```python
from build123d import *

# Parameters (mm, degrees)
F1_DEPTH = 38.09291
F3_DEPTH = 122.48907
F6_W     = 30.103382
F6_H     = 15.981055
F7_DEPTH = 76.09144


with BuildPart() as f1:
    # F0 (on Top) → F1 (new body)
    with BuildSketch(Plane.XY):
        with BuildLine():
            Line((-47.8804, 57.96845), (-61.8804, 57.96845))
            ThreePointArc((-61.8804, 57.96845), (-64.00172, 57.089771), (-64.8804, 54.96845))
            Line((-64.8804, 54.96845), (-64.8804, -39.03155))
            ThreePointArc((-64.8804, -39.03155), (-64.00172, -41.15287), (-61.8804, -42.03155))
            Line((-61.8804, -42.03155), (32.1196, -42.03155))
            ThreePointArc((32.1196, -42.03155), (34.240921, -41.15287), (35.1196, -39.03155))
            Line((35.1196, -39.03155), (35.1196, 54.96845))
            ThreePointArc((35.1196, 54.96845), (34.240921, 57.089771), (32.1196, 57.96845))
            Line((32.1196, 57.96845), (18.1196, 57.96845))
            ThreePointArc((18.1196, 57.96845), (15.99828, 57.089771), (15.1196, 54.96845))
            Line((15.1196, 54.96845), (15.1196, -22.569584))
            Line((15.1196, -22.569584), (-44.8804, -22.569584))
            Line((-44.8804, -22.569584), (-44.8804, 54.96845))
            ThreePointArc((-44.8804, 54.96845), (-45.759079, 57.089771), (-47.8804, 57.96845))
        make_face()
    extrude(amount=F1_DEPTH)


with BuildPart() as f3:
    # F2 (on Right) → F3 (new body)
    with BuildSketch(Plane.YZ):
        Polygon((-71.411475, 51.98656), (-86.8368, 51.98656), (-102.24022, 16.366137), (-86.814895, 16.366137), align=None)
    extrude(amount=F3_DEPTH)


with BuildPart() as f3_1:
    # F4: moved
    add(f3.part.moved(Location((-76.72278, 70.50282, 2.4462))))


with BuildPart() as f1_1:
    add(f1.part)

    # F5: cut F3
    add(f3_1.part, mode=Mode.SUBTRACT)


with BuildPart() as f7:
    # F6 (on Right) → F7 (new body, symmetric)
    with BuildSketch(Plane.YZ):
        with Locations((-78.402916, 34.753974)):
            Rectangle(F6_W, F6_H)
    extrude(amount=F7_DEPTH, both=True)


with BuildPart() as f7_1:
    # F8: moved
    add(f7.part.moved(Location((0, 44.64814, 0))))


with BuildPart() as f1_2:
    add(f1_1.part)

    # F9: cut F7
    add(f7_1.part, mode=Mode.SUBTRACT)


solid = f1_2.part
```
Work out the finished part from the listing and answer in its coordinate system (mm). A direction names the side the tool comes from. Coordinates: 2 decimals unless noted, no trailing zeros. Write each loop counter-clockwise with the first axis right and the second up, starting at its lowest first coordinate (ties: lowest second). Pieces come first, ordered by that corner, then holes. Notation, with made-up numbers: (52.5, 89) - (77.5, 89) arc R24 ccw to (77.5, 119) - close; hole circle Ø7 at (47, 83.5). An arc over 180 degrees is marked (long way). Answer as a JSON object with one key per item and string values.
Q1. Consider L1, parallel to X at y = 9.5, z = 15.5; L2, parallel to Y at x = -22, z = 7; L3, parallel to Y at x = 30, z = 26.5. Determine where each line is inside the solid, lowest interval first. Write a range as from..to.
Results list:
{"L1": "x = -64.88..-44.88, 15.12..35.12", "L2": "y = -42.03..-22.57", "L3": "y = -42.03..-28.41, -12.99..57.97"}
Q2. Given pin 1 Ø7 at (x, y) = (1.5, -37.5) entering from +Z; pin 2 Ø8 at (x, z) = (9, 12) entering from +Y, each flat-ended and moving along its own axis, determine where each tip first touches the part or whether it passes through.
Results list:
{"pin 1": "stops at z = 26.76", "pin 2": "stops at y = -22.57"}
Q3. Find section B-B (z = 20). Write down the section's boundary in (x, y), plus the area to 3 significant figures.
Results list:
{"outline": "(-64.88, -39.03) arc R3 ccw to (-61.88, -42.03) - (32.12, -42.03) arc R3 ccw to (35.12, -39.03) - (35.12, -31.22) - (-64.88, -31.22) - close; (-64.88, -15.8) - (-44.88, -15.8) - (-44.88, 54.97) arc R3 ccw to (-47.88, 57.97) - (-61.88, 57.97) arc R3 ccw to (-64.88, 54.97) - close; (15.12, -15.8) - (35.12, -15.8) - (35.12, 54.97) arc R3 ccw to (32.12, 57.97) - (18.12, 57.97) arc R3 ccw to (15.12, 54.97) - close", "area": "4,020 mm^2"}
Q4. For a pull along X with two mould halves and no side action, classify faces 4 (the flat face through (-44.88, 16, 19)), 5 (the flat face through (-64.88, 9, 19)), 6 (the flat face through (35.12, 7, 19)), 7 (the flat face through (-55, 57.968, 19)) as pulls with the +X half, pulls with the -X half, needs draft (parallel to the pull), parting line crosses it, or undercut.
Results list:
{"face 4": "undercut", "face 5": "pulls with the -X half", "face 6": "pulls with the +X half", "face 7": "needs draft"}
Q5. Which of the six approach directions +Z, -Z, +X, -X, +Y, -Y give full straight-line access (tool end or side, diameter ignored) to faces 1 (the flat face through (-15.58, -29.994, 22.844)), 2 (the flat face through (-14, -22.57, 9)), 3 (the flat face through (-14, -35, 26.763))?
Results list:
{"face 1": "+X, -X", "face 2": "+Z, -Z, +Y", "face 3": "+Z, +X, -X, -Y"}
Q6. Find section A-A (y = -21). Write down the section's boundary in (x, z).
Results list:
{"outline": "(-64.88, 0) - (-44.88, 0) - (-44.88, 18.81) - (-64.88, 18.81) - close; (15.12, 0) - (35.12, 0) - (35.12, 18.81) - (15.12, 18.81) - close"}
Q7. Find section D-D (y = 2.5). Write down the section's boundary in (x, z), plus the area to 3 significant figures.
Results list:
{"outline": "(-64.88, 0) - (-44.88, 0) - (-44.88, 38.09) - (-64.88, 38.09) - close; (15.12, 0) - (35.12, 0) - (35.12, 38.09) - (15.12, 38.09) - close", "area": "1,520 mm^2"}
Q8. Find section C-C (z = 32). Write down the section's boundary in (x, y).
Results list:
{"outline": "(-64.88, -10.61) - (-44.88, -10.61) - (-44.88, 54.97) arc R3 ccw to (-47.88, 57.97) - (-61.88, 57.97) arc R3 ccw to (-64.88, 54.97) - close; (15.12, -10.61) - (35.12, -10.61) - (35.12, 54.97) arc R3 ccw to (32.12, 57.97) - (18.12, 57.97) arc R3 ccw to (15.12, 54.97) - close"}
